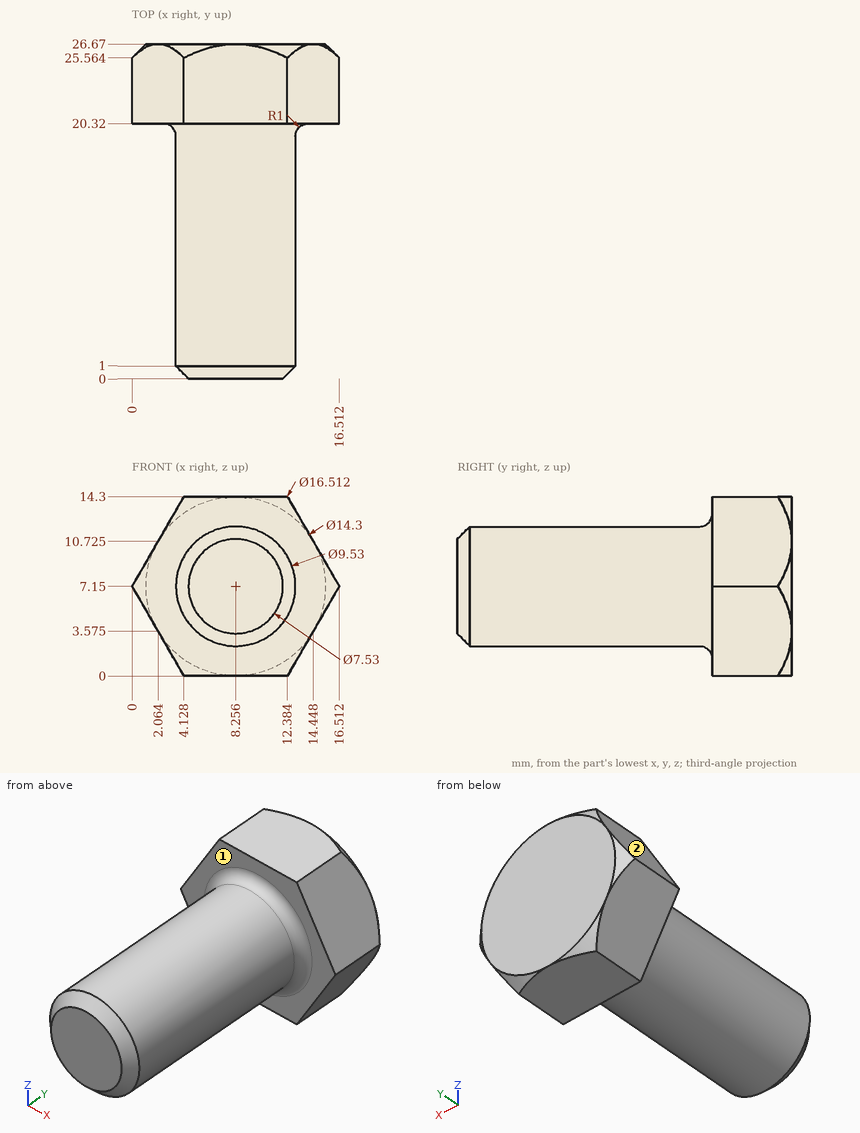
The figure shows three views and two pictorial views of one solid part (mm, origin at its lowest corner). Answer the questions. A direction names the side the tool comes from. Round coordinates to 2 decimals unless told otherwise and drop trailing zeros. Write each question's results on one line, items separated by ' | '.
Q1. Which of the six approach directions +Z, -Z, +X, -X, +Y, -Y give full straight-line access (tool end or side, diameter ignored) to the marked faces 1 and 2?
Data:
face 1: -Y | face 2: +Z, -X, +Y, -Y
Q2. Flat-ended cylindrical pins translate along their axes: P1, Ø3, axis at y = 9, z = 3.5, coming from the +X side; P2, Ø4, axis at x = 10.5, y = 11, coming from the -Z side; P3, Ø8, axis at x = 9.5, y = 14.5, coming from the +Z side (3 decimals). Find the tip coordinate at first contact, or state that the pin passes through.
Data:
P1: x = 12.51 | P2: z = 2.39 | P3: z = 11.915
Q3. Straight lines are drawn through the part: line 1 along Y through (x, z) = (3, 2.5); line 2 along Z through (x, y) = (8, 14.75); line 3 along X through (y, z) = (20, 8.5) (1 decimal). For each, find the intervals that lie inside material, in ascending order. Write a range as [from, to].
Data:
line 1: [20.32, 26.67] | line 2: [2.39, 11.91] | line 3: [3.4, 13.1]
